The model under review builds one solid part; all positions refer to its coordinate system, in mm. A direction names the side the tool comes from. Round coordinates to 2 decimals unless told otherwise and drop trailing zeros. Order: outer loops, then holes, each group sorted by start corner. A loop starts at its lowest first (then second) coordinate and runs counter-clockwise, first axis right, second up.
1) Consider section A-A (y = 5). Give the boundary of the cut face in (x, z), then the cut area to 3 significant figures.
2) Mouldability with a two-part tool opening along X and no side actions: class faces 4 (the face through (38.715, -2.699, 1.014)), 5 (the face through (5, -3, 1)), 6 (the face through (10, -1.5, 1)), 7 (the face through (0.285, 6.599, 1.014)) as pulls with the +X half, pulls with the -X half, needs draft (parallel to the pull), parting line crosses it, or undercut.
3) Consider section D-D (z = 8.25). Give the boundary of the cut face in (x, y), then the cut area to 3 significant figures.
4) Consider section C-C (z = 1). Give the boundary of the cut face in (x, y), then the cut area to 3 significant figures.
5) To check wall thickness, follow L1, parallel to X at y = 3.7, z = 7; L2, parallel to Z at x = 9.5, y = 2.7; L3, parallel to X at y = 4.75, z = 6. State the ranges of each line that lie inside material, in increasing order.
6) Consider section B-B (x = 36). Give the boundary of the cut face in (y, z).
7) Clearance check with flat-ended pins moving along their axes: P1, Ø2.5, axis at x = 11, z = 6, coming from the +Y side; P2, Ø0.7, axis at x = 15.5, y = 6.5, coming from the +Z side; P3, Ø3, axis at x = 9, z = 3, coming from the -Y side; P4, Ø5, axis at x = 27, z = 7.5, coming from the -Y side. State where each tip first meets the part, or that it passes through.
8) Machinability: for faces 1 (the face through (20, 6, 2)), 2 (the face through (29, -1.5, 1)), 3 (the face through (19, 1.65, 6)), which of the approach directions +Z, -Z, +X, -X, +Y, -Y give a long, thin tool a straight path to every point of the face, cutting with its end or side? Answer none if there is none.
from build123d import *

# Parameters (mm, degrees)
BOSS_EXTRU_1_DEPTH           = 2
ESQUISSE2_W                  = 39
ESQUISSE2_H                  = 3.8
BOSS_EXTRU_2_DEPTH           = 8
ENL_V_MAT_EXTRU_1_DEPTH      = 41.602493766
ENL_V_MAT_EXTRU_1_DEPTH_BACK = 41.602493766
ESQUISSE3_R                  = 2
CONG_1_R                     = 1


with BuildPart() as part:
    # Esquisse1 → Boss.-Extru.1 (new body)
    with BuildSketch(Plane.XY):
        Polygon((0, 0), (0, 6.9), (39, 6.9), (39, 0), (39, -3), (29, -3), (29, 0), (10, 0), (10, -3), (0, -3), align=None)
    extrude(amount=BOSS_EXTRU_1_DEPTH)

    # Esquisse2 → Boss.-Extru.2 (add)
    with BuildSketch(Plane.XY.offset(2)):
        with Locations((19.5, 3.55)):
            Rectangle(ESQUISSE2_W, ESQUISSE2_H)
    extrude(amount=BOSS_EXTRU_2_DEPTH)

    # Esquisse3 → Enlèv. mat.-Extru.1 (cut, two sides: drawn at the far end of the back side and taken through both)
    with BuildSketch(Plane(origin=(0, 1.65, 0), x_dir=(1, 0, 0), z_dir=(0, 1, 0)).offset(-ENL_V_MAT_EXTRU_1_DEPTH_BACK)):
        with Locations(Location((9.5, -7, 0), (0, 0, 180))):
            Circle(ESQUISSE3_R)
        with Locations(Location((29.5, -7, 0), (0, 0, 180))):
            Circle(ESQUISSE3_R)
    extrude(amount=ENL_V_MAT_EXTRU_1_DEPTH + ENL_V_MAT_EXTRU_1_DEPTH_BACK, mode=Mode.SUBTRACT)

    # Congé1
    cong_1_edges = [part.edges().sort_by_distance(p)[0] for p in [
        (0, 6.9, 1),
        (39, 6.9, 1),
        (39, -3, 1),
        (29, -3, 1),
        (29, 0, 1),
        (10, 0, 1),
        (10, -3, 1),
        (0, -3, 1),
    ]]
    fillet(cong_1_edges, radius=CONG_1_R)


solid = part.part
Answer below:
1. outline: (0, 0) - (39, 0) - (39, 10) - (0, 10) - close; hole circle Ø4 at (9.5, 7); hole circle Ø4 at (29.5, 7)
1. area: 365 mm2
2. face 4: pulls with the +X half
2. face 5: needs draft
2. face 6: undercut
2. face 7: pulls with the -X half
3. outline: (0, 1.65) - (7.94, 1.65) - (7.94, 5.45) - (0, 5.45) - close; (11.06, 1.65) - (27.94, 1.65) - (27.94, 5.45) - (11.06, 5.45) - close; (31.06, 1.65) - (39, 1.65) - (39, 5.45) - (31.06, 5.45) - close
3. area: 124 mm2
4. outline: (0, -2) arc R1 ccw to (1, -3) - (9, -3) arc R1 ccw to (10, -2) - (10, -1) arc R1 cw to (11, 0) - (28, 0) arc R1 cw to (29, -1) - (29, -2) arc R1 ccw to (30, -3) - (38, -3) arc R1 ccw to (39, -2) - (39, 5.9) arc R1 ccw to (38, 6.9) - (1, 6.9) arc R1 ccw to (0, 5.9) - close
4. area: 328 mm2
5. L1: x = 0 to 7.5, 11.5 to 27.5, 31.5 to 39
5. L2: z = 0 to 5, 9 to 10
5. L3: x = 0 to 7.77, 11.23 to 27.77, 31.23 to 39
6. outline: (-3, 0) - (6.9, 0) - (6.9, 2) - (5.45, 2) - (5.45, 10) - (1.65, 10) - (1.65, 2) - (-3, 2) - close
7. P1: stops at y = 5.45
7. P2: stops at z = 2
7. P3: stops at y = -3
7. P4: stops at y = 1.65
8. face 1: +Z, +X, -X, +Y
8. face 2: +Z, -Z, -Y
8. face 3: +Z, +X, -X, -Y
